Input: part model. Units: mm. Frame: model coordinates. Face numbers are marked on the shaded views. A direction names the side the tool comes from. Give positions to 0.01 mm unless a question says otherwise; leave off trailing zeros. Loops run counter-clockwise (first coordinate to the right, second up) from the corner with the lowest first, then second, coordinate; pieces in that order, holes last. Notation, with made-up numbers: (75.25, -11.5) - (104.25, -11.5) arc R15 cw to (104.25, -6.5) - close; hole circle Ø8 at (17, 47.5). An arc over 180 degrees is marked (long way). Answer as a JSON object with one key per item and string values.
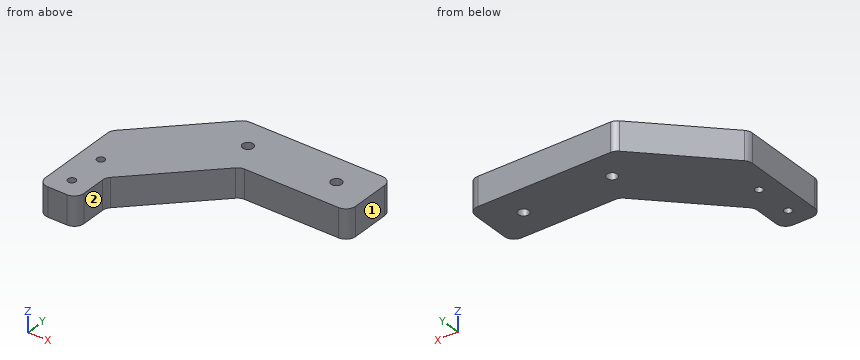
from build123d import *

# Parameters (mm, degrees)
BOSS_EXTRUDE1_DEPTH = 15
CUT_EXTRUDE3_REACH  = 133.457
SKETCH2_R           = 2
SKETCH2_R_2         = 2.75
CHAMFER1_SIZE       = 40
FILLET1_R           = 5


with BuildPart() as part:
    # Sketch1 → Boss-Extrude1 (new body)
    with BuildSketch(Plane.XY):
        Polygon((0, -60), (0, 30), (116, 30), (116, 0), (20, 0), (20, -60), align=None)
    extrude(amount=BOSS_EXTRUDE1_DEPTH)

    # Sketch2 → Cut-Extrude3 (cut, up to next)
    with BuildSketch(Plane.XY, mode=Mode.PRIVATE) as cut_extrude3_sk1:
        with Locations(Location((10, -50, 0), (0, 0, 180))):
            Circle(SKETCH2_R)
    cut_extrude3_tool1 = extrude(cut_extrude3_sk1.sketch, amount=CUT_EXTRUDE3_REACH, mode=Mode.PRIVATE) & part.part
    # Sketch2 → Cut-Extrude3 (cut, up to next)
    with BuildSketch(Plane.XY, mode=Mode.PRIVATE) as cut_extrude3_sk2:
        with Locations(Location((10, -30, 0), (0, 0, 180))):
            Circle(SKETCH2_R)
    cut_extrude3_tool2 = extrude(cut_extrude3_sk2.sketch, amount=CUT_EXTRUDE3_REACH, mode=Mode.PRIVATE) & part.part
    # Sketch2 → Cut-Extrude3 (cut, up to next)
    with BuildSketch(Plane.XY, mode=Mode.PRIVATE) as cut_extrude3_sk3:
        with Locations(Location((52.5, 15, 0), (0, 0, 180))):
            Circle(SKETCH2_R_2)
    cut_extrude3_tool3 = extrude(cut_extrude3_sk3.sketch, amount=CUT_EXTRUDE3_REACH, mode=Mode.PRIVATE) & part.part
    # Sketch2 → Cut-Extrude3 (cut, up to next)
    with BuildSketch(Plane.XY, mode=Mode.PRIVATE) as cut_extrude3_sk4:
        with Locations(Location((98.5, 15, 0), (0, 0, 180))):
            Circle(SKETCH2_R_2)
    cut_extrude3_tool4 = extrude(cut_extrude3_sk4.sketch, amount=CUT_EXTRUDE3_REACH, mode=Mode.PRIVATE) & part.part
    add(cut_extrude3_tool1.solids().sort_by_distance((10, -50, 0))[0], mode=Mode.SUBTRACT)
    add(cut_extrude3_tool2.solids().sort_by_distance((10, -30, 0))[0], mode=Mode.SUBTRACT)
    add(cut_extrude3_tool3.solids().sort_by_distance((52.5, 15, 0))[0], mode=Mode.SUBTRACT)
    add(cut_extrude3_tool4.solids().sort_by_distance((98.5, 15, 0))[0], mode=Mode.SUBTRACT)

    # Chamfer1
    chamfer1_edges = [part.edges().sort_by_distance(p)[0] for p in [
        (0, 30, 7.5),
        (20, 0, 7.5),
    ]]
    chamfer(chamfer1_edges, length=CHAMFER1_SIZE)

    # Fillet1
    fillet1_edges = [part.edges().sort_by_distance(p)[0] for p in [
        (0, -60, 7.5),
        (116, 30, 7.5),
        (116, 0, 7.5),
        (20, -60, 7.5),
        (0, -10, 7.5),
        (40, 30, 7.5),
        (60, 0, 7.5),
        (20, -40, 7.5),
    ]]
    fillet(fillet1_edges, radius=FILLET1_R)


solid = part.part
Item 1: Cut plane D-D (y = 15). Return loops of the section in (x, z).
Geometry check:
{"outline": "(25, 0) - (49.75, 0) - (49.75, 15) - (25, 15) - close; (55.25, 0) - (95.75, 0) - (95.75, 15) - (55.25, 15) - close; (101.25, 0) - (116, 0) - (116, 15) - (101.25, 15) - close"}
Item 2: Cut plane C-C (z = 12). Return loops of the section in (x, y), then the cut area to 3 significant figures.
Geometry check:
{"outline": "(0, -55) arc R5 ccw to (5, -60) - (15, -60) arc R5 ccw to (20, -55) - (20, -42.07) arc R5 cw to (21.46, -38.54) - (58.54, -1.46) arc R5 cw to (62.07, 0) - (111, 0) arc R5 ccw to (116, 5) - (116, 25) arc R5 ccw to (111, 30) - (42.07, 30) arc R5 ccw to (38.54, 28.54) - (1.46, -8.54) arc R5 ccw to (0, -12.07) - close; hole circle Ø4 at (10, -50); hole circle Ø4 at (10, -30); hole circle Ø5.5 at (52.5, 15); hole circle Ø5.5 at (98.5, 15)", "area": "4,590 mm2"}
Item 3: Material intervals for line 1 (Y direction, x = 10, z = 12); line 2 (X direction, y = 15, z = 6.75); line 3 (X direction, y = -30, z = 9.75), sorted ascending. Write a range as [from, to].
Geometry check:
{"line 1": "y = [-60, -52], [-48, -32], [-28, 0]", "line 2": "x = [25, 49.75], [55.25, 95.75], [101.25, 116]", "line 3": "x = [0, 8], [12, 30]"}
Item 4: Cut plane A-A (x = 52.5). Return loops of the section in (y, z).
Geometry check:
{"outline": "(-7.5, 0) - (12.25, 0) - (12.25, 15) - (-7.5, 15) - close; (17.75, 0) - (30, 0) - (30, 15) - (17.75, 15) - close"}
Item 5: Contact query for flat-ended pins moving along their axis: P1, Ø6, axis at y = -10.5, z = 9.5, coming from the +X side; P2, Ø2.5, axis at x = 10, y = -50, coming from the +Z side; P3, Ø6.5, axis at y = -49.5, z = 8, coming from the +X side; P4, Ø4.5, axis at x = 84.5, z = 4, coming from the -Y side. Output: stop coordinate, or through.
Geometry check:
{"P1": "stops at x = 52.5", "P2": "passes through", "P3": "stops at x = 20", "P4": "stops at y = 0"}
Item 6: Cut plane B-B (y = -50). Return loops of the section in (x, z), then the cut area to 3 significant figures.
Geometry check:
{"outline": "(0, 0) - (8, 0) - (8, 15) - (0, 15) - close; (12, 0) - (20, 0) - (20, 15) - (12, 15) - close", "area": "240 mm2"}
Item 7: Access query for the marked faces 1 and 2. Directions: +Z, -Z, +X, -X, +Y, -Y. A direction counts if a zero-diameter tool reaches every point of the face in a straight line with its end or side. Return the directions, or none.
Geometry check:
{"face 1": "+Z, -Z, +X, +Y, -Y", "face 2": "+Z, -Z, +X, -Y"}
